Read the model definition and answer for the solid it produces. Units are mm, in the model's axes. A direction names the side the tool comes from. Give positions to 0.01 mm unless a question says otherwise; leave off trailing zeros. Write each loop counter-clockwise with the first axis right and the second up, starting at its lowest first coordinate (ties: lowest second). Pieces come first, ordered by that corner, then holes. Notation, with made-up numbers: (63, 47) - (99, 47) arc R24 ccw to (99, 61) - close; hole circle Ø8 at (-21, 84). An arc over 180 degrees is marked (long way). Answer as a JSON object with one key per item and string values. Group by question number.
```python
from build123d import *

# Parameters (mm, degrees)
RESSALTO_EXTRUS_O1_DEPTH = 200


with BuildPart() as part:
    # Esboço1 → Ressalto-extrusão1 (new body)
    with BuildSketch(Plane(origin=(0, 0, 0), x_dir=(1, 0, 0), z_dir=(0, 1, 0))):
        with BuildLine():
            Line((-3.25, -0.34285984), (3.25, -0.34285984))
            Line((3.25, -0.34285984), (3.25, 9.45714016))
            ThreePointArc((3.25, 9.45714016), (9.993573839, 0.358443767), (3.919183588, -9.2))
            ThreePointArc((3.919183588, -9.2), (0, -6), (-3.919183588, -9.2))
            ThreePointArc((-3.919183588, -9.2), (-9.993573839, 0.358443767), (-3.25, 9.45714016))
            Line((-3.25, 9.45714016), (-3.25, -0.34285984))
        make_face()
    extrude(amount=RESSALTO_EXTRUS_O1_DEPTH)


solid = part.part
```
1) Find section D-D, the plane x = -7.25. Write down the section's boundary in (y, z).
2) For a pull along X with two mould halves and no side action, classify faces 1 (the cylindrical face through (-10, 99, 0)), 2 (the flat face through (0, 0, 2)), 3 (the flat face through (-3.25, 99, -5)) as released by +X, released by -X, zero draft, split by the parting line, or undercut.
3) Find section C-C, the plane x = 8. Write down the section's boundary in (y, z).
4) Flat-ended cylindrical pins translate along their axes: pin 1 Ø2 at (y, z) = (44, 7) entering from +X; pin 2 Ø1 at (y, z) = (73, -7) entering from +X; pin 3 Ø8 at (y, z) = (105, -5.5) entering from -X. Find the tip coordinate at first contact, or state that the pin passes through.
5) Find the intervals of material crossed by line 1 (X direction, y = 27, z = 0.25); line 2 (Z direction, x = 0.5, y = 151.5); line 3 (X direction, y = 164.5, z = -7.5), in increasing order. Write a range as [from, to].
6) Find section A-A, the plane z = -6.5. Write down the section's boundary in (x, y), and give its area (3 significant figures).
7) Find section B-B, the plane y = 36. Write down the section's boundary in (x, z), and give its area (3 significant figures).
8) Which of the six approach directions +Z, -Z, +X, -X, +Y, -Y give full straight-line access (tool end or side, diameter ignored) to faces 4 (the flat face through (0, 99, 0.343)), 5 (the flat face through (0, 200, 2))?
Values follow:
{
 "1": {"outline": "(0, -6.89) - (200, -6.89) - (200, 6.89) - (0, 6.89) - close"},
 "2": {"face 1": "released by -X", "face 2": "zero draft", "face 3": "undercut"},
 "3": {"outline": "(0, -6) - (200, -6) - (200, 6) - (0, 6) - close"},
 "4": {"pin 1": "stops at x = 8", "pin 2": "stops at x = 7.6", "pin 3": "stops at x = -9.89"},
 "5": {"line 1": "x = [-10, -3.25], [3.25, 10]", "line 2": "z = [0.34, 6.03]", "line 3": "x = [-6.61, -3.25], [3.25, 6.61]"},
 "6": {"outline": "(-7.6, 0) - (-3.25, 0) - (-3.25, 200) - (-7.6, 200) - close; (3.25, 0) - (7.6, 0) - (7.6, 200) - (3.25, 200) - close", "area": "1,740 mm2"},
 "7": {"outline": "(-3.92, 9.2) arc R10 ccw to (-3.25, -9.46) - (-3.25, 0.34) - (3.25, 0.34) - (3.25, -9.46) arc R10 ccw to (3.92, 9.2) arc R4 cw to start", "area": "225 mm2"},
 "8": {"face 4": "-Z, +Y, -Y", "face 5": "+Z, -Z, +X, -X, +Y"}
}
